from build123d import *

# Parameters (mm, degrees)
SKETCH1_W               = 1.5
SKETCH1_H               = 33.5
SKETCH1_W_2             = 33.5
SKETCH1_H_2             = 1.5
BOSS_EXTRUDE1_DEPTH     = 210
CUT_EXTRUDE7_DEPTH      = 81
CUT_EXTRUDE7_DEPTH_BACK = 52
CUT_EXTRUDE8_DEPTH      = 52
CUT_EXTRUDE8_DEPTH_BACK = 52
SKETCH5_R               = 2.75
CUT_EXTRUDE9_DEPTH      = 52
SKETCH6_R               = 2.75
CUT_EXTRUDE10_DEPTH     = 52


with BuildPart() as part:
    # Sketch1 → Boss-Extrude1 (new body)
    with BuildSketch(Plane.XY):
        with Locations((0, 0.75)):
            Rectangle(SKETCH1_W, SKETCH1_H)
        with Locations((17.5, -16.75)):
            Rectangle(SKETCH1_W_2, SKETCH1_H_2)
        with Locations((0, -16.75)):
            Rectangle(SKETCH1_W, SKETCH1_H_2)
    extrude(amount=BOSS_EXTRUDE1_DEPTH)

    # Sketch2 → Cut-Extrude7 (cut, two sides)
    with BuildSketch(Plane(origin=(0, -16, 0), x_dir=(1, 0, 0), z_dir=(0, 1, 0))) as cut_extrude7_sk:
        Polygon((0.75, -16.061643836), (17.5, 0), (0.75, 0), align=None)
        Polygon((0.75, -56), (0.75, -16.061643836), (0.75, 0), (-0.75, 0), (-0.75, -17.5), (-0.75, -56), align=None)
        Polygon((34.25, -210), (34.25, -140), (16.75, -140), (0.75, -157), (0.75, -210), align=None)
    extrude(amount=CUT_EXTRUDE7_DEPTH, mode=Mode.SUBTRACT)
    extrude(cut_extrude7_sk.sketch, amount=-CUT_EXTRUDE7_DEPTH_BACK, mode=Mode.SUBTRACT)

    # Sketch4 → Cut-Extrude8 (cut, two sides)
    with BuildSketch(Plane(origin=(0.75, 0, 0), x_dir=(0, 0, -1), z_dir=(1, 0, 0))) as cut_extrude8_sk:
        Polygon((-73.5, 1.5), (-56, -16), (-56, 17.5), (-73.5, 17.5), align=None)
        Polygon((-210, 0), (-192.5, -17.5), (-210, -17.5), align=None)
    extrude(amount=CUT_EXTRUDE8_DEPTH, mode=Mode.SUBTRACT)
    extrude(cut_extrude8_sk.sketch, amount=-CUT_EXTRUDE8_DEPTH_BACK, mode=Mode.SUBTRACT)

    # Sketch5 → Cut-Extrude9 (cut)
    with BuildSketch(Plane(origin=(0.75, 0, 0), x_dir=(0, 0, -1), z_dir=(1, 0, 0))):
        with Locations((-72, -5.5)):
            Circle(SKETCH5_R)
        with Locations((-92, -5.5)):
            Circle(SKETCH5_R)
        with Locations((-112, -5.5)):
            Circle(SKETCH5_R)
        with Locations((-132, -5.5)):
            Circle(SKETCH5_R)
        with Locations((-152, -5.5)):
            Circle(SKETCH5_R)
        with Locations((-172, -5.5)):
            Circle(SKETCH5_R)
        with Locations((-192, -5.5)):
            Circle(SKETCH5_R)
        with Locations((-202, 9.5)):
            Circle(SKETCH5_R)
        with Locations((-182, 9.5)):
            Circle(SKETCH5_R)
        with Locations((-162, 9.5)):
            Circle(SKETCH5_R)
        with Locations((-142, 9.5)):
            Circle(SKETCH5_R)
        with Locations((-122, 9.5)):
            Circle(SKETCH5_R)
        with Locations((-102, 9.5)):
            Circle(SKETCH5_R)
        with Locations((-82, 9.5)):
            Circle(SKETCH5_R)
    extrude(amount=-CUT_EXTRUDE9_DEPTH, mode=Mode.SUBTRACT)

    # Sketch6 → Cut-Extrude10 (cut)
    with BuildSketch(Plane(origin=(0, -16, 0), x_dir=(1, 0, 0), z_dir=(0, 1, 0))):
        with Locations((26.25, -8)):
            Circle(SKETCH6_R)
        with Locations((26.25, -28)):
            Circle(SKETCH6_R)
        with Locations((26.25, -48)):
            Circle(SKETCH6_R)
        with Locations((26.25, -68)):
            Circle(SKETCH6_R)
        with Locations((26.25, -88)):
            Circle(SKETCH6_R)
        with Locations((26.25, -108)):
            Circle(SKETCH6_R)
        with Locations((26.25, -128)):
            Circle(SKETCH6_R)
        with Locations((11.25, -138)):
            Circle(SKETCH6_R)
        with Locations((11.25, -118)):
            Circle(SKETCH6_R)
        with Locations((11.25, -98)):
            Circle(SKETCH6_R)
        with Locations((11.25, -78)):
            Circle(SKETCH6_R)
        with Locations((11.25, -58)):
            Circle(SKETCH6_R)
        with Locations((11.25, -38)):
            Circle(SKETCH6_R)
        with Locations((11.25, -18)):
            Circle(SKETCH6_R)
    extrude(amount=-CUT_EXTRUDE10_DEPTH, mode=Mode.SUBTRACT)


solid = part.part
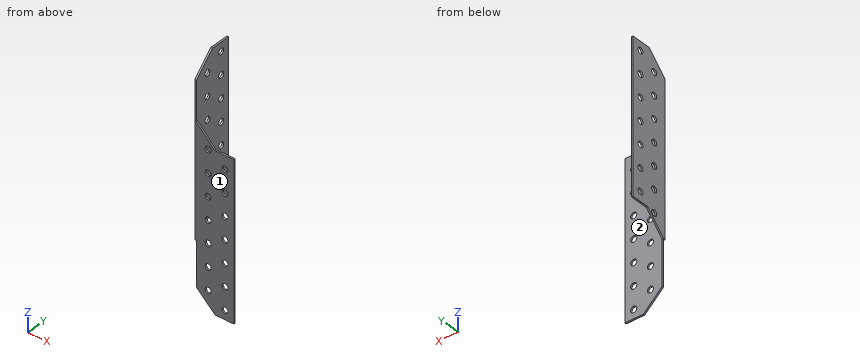
Could you check a few things on this model? Use its own coordinates, in mm. Face numbers are marked on the shaded views. A direction names the side the tool comes from. Give positions to 0.01 mm unless a question says otherwise; leave off trailing zeros. Loops run counter-clockwise (first coordinate to the right, second up) from the corner with the lowest first, then second, coordinate; pieces in that order, holes last. Notation, with made-up numbers: (29, -10.75) -> (79, -10.75) arc R22 ccw to (79, -4.75) -> close; hole circle Ø6 at (49, 23). An arc over 180 degrees is marked (long way). Answer as CSV lines item,"result". Start each with the question number.
(1) If we section it at C-C on z = 8: Write out the boundary of the cut face in (x, y), then the cut area to 3 significant figures.
(2) If we section it at B-B on x = 21: Write out the boundary of the cut face in (y, z), then the cut area to 3 significant figures.
(3) If we section it at A-A on z = 162: Write out the boundary of the cut face in (x, y), then the cut area to 4 significant figures.
(4) I'm going to push flat-ended pins straight in: pin 1 Ø6.5 at (x, z) = (11.25, 118) entering from -Y; pin 2 Ø0.8 at (x, y) = (27, -17) entering from +Z; pin 3 Ø0.8 at (x, y) = (0, -16.5) entering from -Z; pin 4 Ø9 at (x, z) = (26.25, 48) entering from +Y. Where does each tip first touch, or does it pass through?
(5) If we section it at D-D on y = 5: Write out the boundary of the cut face in (x, z), then the cut area to 3 significant figures.
(6) Which directions (+Z, -Z, +X, -X, +Y, -Y) give clear straight access to the entire face, cutting with the end or side of a thin tool? Please do the marked faces 1 and 2.
(7) I need wall thicknesses on probe 1 along Y at (x, z) = (0, 92); probe 2 along X at (y, z) = (-16.75, 108); probe 3 along Y at (x, z) = (24, 103). Which ranges of each line are inside material? Lowest first, please.
Computed:
1,outline,"(9.16, -17.5) -> (23.5, -17.5) -> (23.5, -16) -> (9.16, -16) -> close; (29, -17.5) -> (34.25, -17.5) -> (34.25, -16) -> (29, -16) -> close"
1,area,"29.4 mm2"
2,outline,"(-17.5, 0) -> (-16, 0) -> (-16, 140) -> (-17.5, 140) -> close"
2,area,"210 mm2"
3,outline,"(-0.75, -17.5) -> (0.75, -17.5) -> (0.75, 6.75) -> (-0.75, 6.75) -> close; (-0.75, 12.25) -> (0.75, 12.25) -> (0.75, 17.5) -> (-0.75, 17.5) -> close"
3,area,"44.25 mm2"
4,pin 1,"stops at y = -17.5"
4,pin 2,"stops at z = 140"
4,pin 3,"stops at z = 56"
4,pin 4,"stops at y = -16"
5,outline,"(-0.75, 73.5) -> (0.75, 73.5) -> (0.75, 210) -> (-0.75, 210) -> close"
5,area,"205 mm2"
6,face 1,"+Z, -Z, +X, -X, -Y"
6,face 2,"+Z, -Z, +X, +Y"
7,probe 1,"y = -17.5 to -8.25, -2.75 to 17.5"
7,probe 2,"x = -0.75 to 23.5, 29 to 34.25"
7,probe 3,"y = -17.5 to -16"
